from build123d import *

# Parameters (mm, degrees)
SKETCH1_W           = 26
SKETCH1_H           = 10
BOSS_EXTRUDE1_DEPTH = 20
SKETCH2_W           = 10
SKETCH2_H           = 21.6
CUT_EXTRUDE1_DEPTH  = 15
SKETCH3_R           = 1.9
CUT_EXTRUDE2_DEPTH  = 0.8


with BuildPart() as part:
    # Sketch1 → Boss-Extrude1 (new body)
    with BuildSketch(Plane(origin=(0, 0, 0), x_dir=(0, 1, 0), z_dir=(0, 0, 1))):
        Rectangle(SKETCH1_W, SKETCH1_H)
    extrude(amount=BOSS_EXTRUDE1_DEPTH)

    # Sketch2 → Cut-Extrude1 (cut)
    with BuildSketch(Plane.XY.offset(20)):
        Rectangle(SKETCH2_W, SKETCH2_H)
    extrude(amount=-CUT_EXTRUDE1_DEPTH, mode=Mode.SUBTRACT)

    # Sketch3 → Cut-Extrude2 (cut)
    with BuildSketch(Plane(origin=(0, -10.8, 0), x_dir=(-1, 0, 0), z_dir=(0, 1, 0))):
        with Locations(Location((0, 14.5, 0), (0, 0, 90))):
            Circle(SKETCH3_R)
    cut_extrude2 = extrude(amount=-CUT_EXTRUDE2_DEPTH, mode=Mode.SUBTRACT)

    # Mirror1: Cut-Extrude2 across plane
    add(cut_extrude2.mirror(Plane.ZX), mode=Mode.SUBTRACT)


solid = part.part
Work out the finished part from the listing and answer in its coordinate system (mm). A direction names the side the tool comes from. Round coordinates to 2 decimals unless told otherwise and drop trailing zeros. Loops run counter-clockwise (first coordinate to the right, second up) from the corner with the lowest first, then second, coordinate; pieces in that order, holes last. Notation, with made-up numbers: (14.25, 2.25) - (47.25, 2.25) arc R5 ccw to (47.25, 6.25) - close; hole circle Ø6 at (-25.5, -17). An arc over 180 degrees is marked (long way). One line per item, written item: value.
Q1. Find section B-B on x = -3.5. Give the vertices of the cut face in (y, z).
Check values:
outline: (-13, 0) - (13, 0) - (13, 20) - (10.8, 20) - (10.8, 5) - (-10.8, 5) - (-10.8, 20) - (-13, 20) - close
Q2. For faces 1 (the flat face through (0, 0, 5)), 2 (the cylindrical face through (0.08, 11.19, 12.6)), 3 (the flat face through (-5, 0, 3)), determine the directions among +Z, -Z, +X, -X, +Y, -Y from which every point of the face is accessible in a straight line to the end or side of a thin tool.
Check values:
face 1: +Z, +X, -X
face 2: none
face 3: +Z, -Z, -X, +Y, -Y
Q3. The mould has two halves that part along X. Classify faces 4 (the flat face through (0, -11.6, 14)), 5 (the flat face through (5, 0, 3)), 6 (the flat face through (-1.2, 10.8, 12.6)): +X half, -X half, draft (parallel to the pull), parting line (faces both ways), or undercut.
Check values:
face 4: undercut
face 5: +X half
face 6: draft
Q4. This flat-tipped pin is pushed along its axis until it touches: pin 1 Ø4 at (x, y) = (3, -8.5) entering from +Z. Where does it stop, or does it pass through?
Check values:
pin 1: z = 5
Q5. Find section D-D on y = -8. Give the vertices of the cut face in (x, z), and give its area (3 significant figures).
Check values:
outline: (-5, 0) - (5, 0) - (5, 5) - (-5, 5) - close
area: 50.0 mm2
Q6. Find section C-C on z = 14.75. Give the vertices of the cut face in (x, y).
Check values:
outline: (-5, -13) - (5, -13) - (5, -10.8) - (1.88, -10.8) - (1.88, -11.6) - (-1.88, -11.6) - (-1.88, -10.8) - (-5, -10.8) - close; (-5, 10.8) - (-1.88, 10.8) - (-1.88, 11.6) - (1.88, 11.6) - (1.88, 10.8) - (5, 10.8) - (5, 13) - (-5, 13) - close
Q7. Find section A-A on z = 5.5. Give the vertices of the cut face in (x, y), and give its area (3 significant figures).
Check values:
outline: (-5, -13) - (5, -13) - (5, -10.8) - (-5, -10.8) - close; (-5, 10.8) - (5, 10.8) - (5, 13) - (-5, 13) - close
area: 44.0 mm2
Q8. Straight lines are drawn through the part: probe 1 along X at (y, z) = (-11, 14.5); probe 2 along Y at (x, z) = (-2, 8.75); probe 3 along Z at (x, y) = (1, -2.75). For each, find the intervals that lie inside material, in ascending order.
Check values:
probe 1: -5 to -1.9, 1.9 to 5
probe 2: -13 to -10.8, 10.8 to 13
probe 3: 0 to 5
